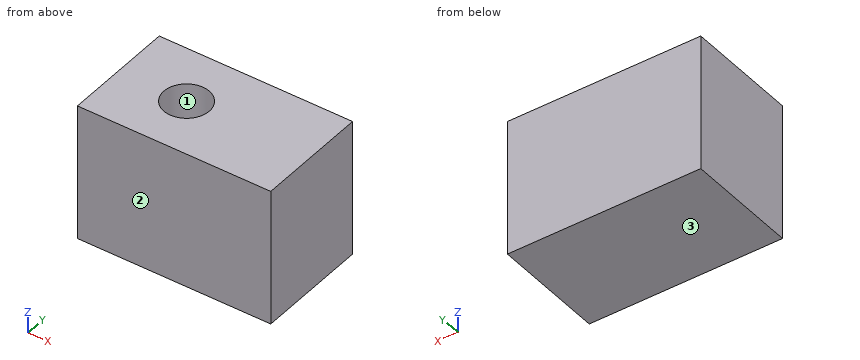
```python
from build123d import *

# Parameters (mm, degrees)
F0_W     = 60
F0_H     = 50
F1_DEPTH = 60
F2_R     = 10
F3_DEPTH = 25
F4_DEPTH = 25


with BuildPart() as f1:
    # F0 (on Top) → F1 (new body)
    with BuildSketch(Plane.XY):
        Rectangle(F0_W, F0_H)
    extrude(amount=F1_DEPTH)

    # F2 (on face) → F3 (cut)
    with BuildSketch(Plane.XY.offset(60)):
        Circle(F2_R)
    extrude(amount=-F3_DEPTH, mode=Mode.SUBTRACT)

    # F4 (add): a face of the model
    f4_faces = [f1.faces().sort_by_distance(p)[0] for p in [
        (30, 0, 30),
    ]]
    extrude(f4_faces, amount=F4_DEPTH)


solid = f1.part
```
Geometry check sheet. Reference: the model listing, model coordinates, mm. Face numbers are marked on the shaded views. Give positions to 0.01 mm unless a question says otherwise; leave off trailing zeros. Loops run counter-clockwise (first coordinate to the right, second up) from the corner with the lowest first, then second, coordinate; pieces in that order, holes last. Notation, with made-up numbers: M -15,66 L 28,66 A26 cw 28,103 Z; hole C 12,75 d5. An arc over 180 degrees is marked long. Write item = value, one per line.
(1) Gauge pin test, flat end, axial feed: pin 1 Ø6 at (x, y) = (-0.5, -1) entering from +Z. Record the tip position at first contact, or that the pin passes through.
Answer below:
pin_1 = 35
(2) Sectioned sample at C-C, the plane z = 37. Record the cut outline in (x, y).
Answer below:
outline = M -30,-25 L 55,-25 L 55,25 L -30,25 Z; hole C 0,0 d20
(3) Release check for a two-part mould opening along Y. For the marked faces 1, 2 and 3 record: released by +Y, released by -Y, zero draft, split by the parting line, or undercut.
Answer below:
face_1 = undercut
face_2 = released by -Y
face_3 = zero draft
(4) Material ranges on line 1 (Y direction, x = 0, z = 54.25); line 2 (Y direction, x = -5.5, z = 38.5); line 3 (X direction, y = -8, z = 45), recorded low to high. Write a range as [from, to].
Answer below:
line_1 = [-25, -10], [10, 25]
line_2 = [-25, -8.35], [8.35, 25]
line_3 = [-30, -6], [6, 55]
(5) Sectioned sample at B-B, the plane y = 0. Record the cut outline in (x, z).
Answer below:
outline = M -30,0 L 55,0 L 55,60 L 10,60 L 10,35 L -10,35 L -10,60 L -30,60 Z
(6) Sectioned sample at A-A, the plane x = 0. Record the cut outline in (y, z).
Answer below:
outline = M -25,0 L 25,0 L 25,60 L 10,60 L 10,35 L -10,35 L -10,60 L -25,60 Z
